For this review, take the finished solid that the model builds, in its own axes (mm). A direction names the side the tool comes from. Coordinates: 2 decimals unless noted, no trailing zeros. Loops run counter-clockwise (first coordinate to the right, second up) from the corner with the lowest first, then second, coordinate; pieces in that order, holes last.
```python
from build123d import *

# Parameters (mm, degrees)
SKETCH3_W           = 192
SKETCH3_H           = 135
BOSS_EXTRUDE1_DEPTH = 5.7
SKETCH9_W           = 115
SKETCH9_H           = 70
CUT_EXTRUDE2_DEPTH  = 47
SKETCH12_R          = 0.5
CUT_EXTRUDE3_DEPTH  = 37
CUT_EXTRUDE4_DEPTH  = 11


with BuildPart() as part:
    # Sketch3 → Boss-Extrude1 (new body)
    with BuildSketch(Plane(origin=(0, 0, 0), x_dir=(1, 0, 0), z_dir=(0, 1, 0))):
        with Locations((90, 53.5)):
            Rectangle(SKETCH3_W, SKETCH3_H)
    extrude(amount=BOSS_EXTRUDE1_DEPTH)

    # Sketch9 → Cut-Extrude2 (cut)
    with BuildSketch(Plane(origin=(0, 0, 0), x_dir=(1, 0, 0), z_dir=(0, 1, 0))):
        with Locations((90, 53)):
            Rectangle(SKETCH9_W, SKETCH9_H)
    extrude(amount=CUT_EXTRUDE2_DEPTH, mode=Mode.SUBTRACT)

    # Sketch12 → Cut-Extrude3 (cut)
    with BuildSketch(Plane(origin=(0, 0, 0), x_dir=(1, 0, 0), z_dir=(0, 1, 0))):
        with Locations((30, 90)):
            Circle(SKETCH12_R)
        with Locations((30, 16)):
            Circle(SKETCH12_R)
        with Locations((150, 16)):
            Circle(SKETCH12_R)
        with Locations((150, 90)):
            Circle(SKETCH12_R)
    extrude(amount=CUT_EXTRUDE3_DEPTH, mode=Mode.SUBTRACT)

    # Sketch13 → Cut-Extrude4 (cut)
    with BuildSketch(Plane(origin=(0, 0, 0), x_dir=(1, 0, 0), z_dir=(0, 1, 0))):
        Polygon((-5.8, 121), (-5.8, 93.9), (0, 93.9), (0, 67.1), (-5.8, 67.1), (-5.8, 39.9), (0, 39.9), (0, 13.1), (-5.8, 13.1), (-5.8, -14), (-9.8, -14), (-9.8, 121), align=None)
        Polygon((189.8, 121), (185.8, 121), (185.8, 93.9), (180, 93.9), (180, 67.1), (185.8, 67.1), (185.8, 39.9), (180, 39.9), (180, 13.1), (185.8, 13.1), (185.8, -14), (189.8, -14), align=None)
    extrude(amount=CUT_EXTRUDE4_DEPTH, mode=Mode.SUBTRACT)


solid = part.part
```
Q1. Machinability: for faces 4 (the face through (-3, 3, -93.9)), 5 (the face through (183, 3, -67.1)), 6 (the face through (89, 3, -18)), which of the approach directions +Z, -Z, +X, -X, +Y, -Y give a long, thin tool a straight path to every point of the face, cutting with its end or side? Answer none if there is none.
Q2. The part is to be moulded in two halves that separate along X. For faces 1 (the face through (0, 3, -27)), 2 (the face through (89, 3, -88)), 3 (the face through (180, 3, -27)), say which applies: +X half, -X half, draft (parallel to the pull), parting line (faces both ways), or undercut.
Q3. Consider section C-C (y = 3.8). State the section outline as (x, z) points.
Q4. For pin 1 Ø3 at (y, z) = (2, -77.5) entering from -X; pin 2 Ø2 at (y, z) = (2.5, -30.5) entering from +X, all flat-tipped, find the tip position at first contact; note any pin that passes through.
Q5. Consider section A-A (z = -48.5). State the section outline as (x, y) points.
Q6. Wall thickness on probe 1 along Z at (x, y) = (30, 3.6); probe 2 along X at (y, z) = (2.5, -90); probe 3 along Z at (x, y) = (68.5, 5.35): over which ranges is each line inside the solid? List them lowest first.
Q7. Consider section B-B (x = 101.5). State the section outline as (y, z) points, then the cut area to 4 significant figures.
Model answer:
1. face 4: -X, +Y, -Y
1. face 5: +X, +Y, -Y
1. face 6: +Y, -Y
2. face 1: -X half
2. face 2: undercut
2. face 3: +X half
3. outline: (-5.8, -121) - (185.8, -121) - (185.8, -93.9) - (180, -93.9) - (180, -67.1) - (185.8, -67.1) - (185.8, -39.9) - (180, -39.9) - (180, -13.1) - (185.8, -13.1) - (185.8, 14) - (-5.8, 14) - (-5.8, -13.1) - (0, -13.1) - (0, -39.9) - (-5.8, -39.9) - (-5.8, -67.1) - (0, -67.1) - (0, -93.9) - (-5.8, -93.9) - close; hole circle Ø1 at (30, -90); hole circle Ø1 at (30, -16); hole (32.5, -88) - (147.5, -88) - (147.5, -18) - (32.5, -18) - close; hole circle Ø1 at (150, -90); hole circle Ø1 at (150, -16)
4. pin 1: stops at x = 0
4. pin 2: stops at x = 180
5. outline: (-5.8, 0) - (32.5, 0) - (32.5, 5.7) - (-5.8, 5.7) - close; (147.5, 0) - (185.8, 0) - (185.8, 5.7) - (147.5, 5.7) - close
6. probe 1: z = -121 to -90.5, -89.5 to -16.5, -15.5 to 14
6. probe 2: x = 0 to 29.5, 30.5 to 149.5, 150.5 to 180
6. probe 3: z = -121 to -88, -18 to 14
7. outline: (0, -121) - (5.7, -121) - (5.7, -88) - (0, -88) - close; (0, -18) - (5.7, -18) - (5.7, 14) - (0, 14) - close
7. area: 370.5 mm2
